```python
from build123d import *

# Parameters (mm, degrees)
F0_W     = 31.75
F0_H     = 19.05
F1_DEPTH = 25.4
F3_D     = 4.7625
F3_DEPTH = 12.7
F3_TIP   = 1.4307993491
F5_D     = 6.35


with BuildPart() as f1:
    # F0 (on Top) → F1 (new body)
    with BuildSketch(Plane.XY):
        with Locations((15.875, 9.525)):
            Rectangle(F0_W, F0_H)
    extrude(amount=F1_DEPTH)

    # F3
    with Locations(Plane(origin=(0, 0, 0), x_dir=(1, 0, 0), z_dir=(0, 0, -1))):
        with Locations((8.041003041, -9.6340968012), (23.916003041, -9.6340968012)):
            Hole(F3_D / 2, depth=F3_DEPTH)
            with Locations((0, 0, -(F3_DEPTH + F3_TIP / 2))):  # 118° drill point
                Cone(0, F3_D / 2, F3_TIP, mode=Mode.SUBTRACT)

    # F5 (through all)
    with Locations(Plane.XZ):
        with Locations((15.875, 17.4625)):
            Hole(F5_D / 2)


solid = f1.part
```
Geometry check sheet. Reference: the model listing, model coordinates, mm. A direction names the side the tool comes from. Round coordinates to 2 decimals unless told otherwise and drop trailing zeros. Loops run counter-clockwise (first coordinate to the right, second up) from the corner with the lowest first, then second, coordinate; pieces in that order, holes last. Notation, with made-up numbers: M 49,-14.5 L 106,-14.5 A22 cw 106,10.5 Z; hole C 38,10.25 d7. An arc over 180 degrees is marked long. Return JSON: item names as keys, results as strings. Group by question number.
(1) Scan lines: line 1 along X through (y, z) = (14.75, 15.5); line 2 along Z through (x, y) = (15, 6); line 3 along X through (y, z) = (10.5, 3.75). Record each from-to range of solid material in increasing order. Write a range as [from, to].
(2) Section check C-C, the plane z = 2.75. Enter the section's corners in (x, y).
(3) Section check A-A, the plane z = 19.5. Enter the section's corners in (x, y), and give its area (3 significant figures).
(4) Set-up check for faces 5 (the face through (16, 0, 13)), 6 (the face through (26.295, 9.529, 6.439)): record each of +Z, -Z, +X, -X, +Y, -Y from which the full face is reachable in a straight line by a thin tool's end or side.
(5) Mould release check, pull along Z, two halves, no side actions. Record for faces 1 (the face through (16, 19.05, 13)), 2 (the face through (14.17, 9.66, 20.14)), 3 (the face through (16, 10, 25.4)), 4 (the face through (23.59, 9.89, 13.88)): pulls with the +Z half, pulls with the -Z half, needs draft (parallel to the pull), parting line crosses it, or undercut.
Data:
{
 "1": {"line 1": "[0, 13.38], [18.37, 31.75]", "line 2": "[0, 14.41], [20.51, 25.4]", "line 3": "[0, 5.82], [10.26, 21.7], [26.13, 31.75]"},
 "2": {"outline": "M 0,0 L 31.75,0 L 31.75,19.05 L 0,19.05 Z; hole C 8.04,9.63 d4.76; hole C 23.92,9.63 d4.76"},
 "3": {"outline": "M 0,0 L 13.44,0 L 13.44,19.05 L 0,19.05 Z; M 18.31,0 L 31.75,0 L 31.75,19.05 L 18.31,19.05 Z", "area": "512 mm²"},
 "4": {"face 5": "+Z, -Z, +X, -X, -Y", "face 6": "-Z"},
 "5": {"face 1": "needs draft", "face 2": "undercut", "face 3": "pulls with the +Z half", "face 4": "pulls with the -Z half"}
}
